Autodesk Inventor part; units mm, degrees
ref_plane "YZ Plane" through (0, 0, 0) normal (1, 0, 0) x (0, 1, 0)
ref_plane "XZ Plane" through (0, 0, 0) normal (0, 1, 0) x (-1, 0, 0)
ref_plane "XY Plane" through (0, 0, 0) normal (0, 0, 1) x (1, 0, 0)
sketch "Sketch1" plane through (0, 0, 0) normal (0, 0, 1) x (1, 0, 0)
  line L0 (0, 0) -> (20, 0)
  line L1 (20, 0) -> (20, 3.2)
  line L2 (0, 3.2) -> (20, 3.2)
  line L3 (0, 0) -> (0, 3.2)
  line L4 (20, -25) -> (0, -25)
  line L5 (0, -25) -> (0, -28.2)
  line L6 (20, -28.2) -> (0, -28.2)
  line L7 (20, -25) -> (20, -28.2)
  line L8 (3.2, -25) -> (3.2, 0)
  line L9 (0, -25) -> (0, 0)
  line L10 (-0.3, -0.3) -> (-0.3, 3.5)
  line L11 (-0.3, 3.5) -> (20.3, 3.5)
  line L12 (20.3, 3.5) -> (20.3, -0.3)
  line L13 (20.3, -24.7) -> (20.3, -28.5)
  line L14 (20.3, -28.5) -> (-0.3, -28.5)
  line L15 (-0.3, -28.5) -> (-0.3, -24.7)
  line L16 (3.5, -24.7) -> (3.5, -0.3)
  line L17 (-0.3, -0.3) -> (-0.3, -24.7)
  line L18 (20.3, -0.3) -> (3.5, -0.3)
  line L19 (3.5, -24.7) -> (20.3, -24.7)
  line L20 (6.5, -3.3) -> (6.5, -21.7)
  line L21 (6.5, -21.7) -> (23.3, -21.7)
  line L22 (23.3, -21.7) -> (23.3, -31.5)
  line L23 (23.3, -31.5) -> (-3.3, -31.5)
  line L24 (-3.3, -31.5) -> (-3.3, -24.7)
  line L25 (-3.3, -24.7) -> (-3.3, -0.3)
  line L26 (-3.3, -0.3) -> (-3.3, 6.5)
  line L27 (-3.3, 6.5) -> (23.3, 6.5)
  line L28 (23.3, 6.5) -> (23.3, -3.3)
  line L29 (23.3, -3.3) -> (6.5, -3.3)
  dimension "d2" = 0.3
  dimension "d3" = 0.3
  dimension "d4" = 0.3
  dimension "d5" = 24.4
  dimension "d6" = 3.8
  dimension "d7" = 3
extrude "Extrusion1" add sketch "Sketch1" against normal blind 15 contours L20 L21 L22 L23 L24 L25 L26 L27 L28 L29
sketch "Sketch4" plane through (0, 0, 0) normal (0, 0, 1) x (1, 0, 0)
  line L0 (23.3, -3.3) -> (23.3, 6.5)
  line L1 (23.3, 6.5) -> (-3.3, 6.5)
  line L2 (23.3, -3.3) -> (6.5, -3.3)
  line L3 (6.5, -3.3) -> (6.5, -21.7)
  line L4 (6.5, -21.7) -> (23.3, -21.7)
  line L5 (-3.3, -0.3) -> (-3.3, 6.5)
  line L6 (-3.3, -31.5) -> (23.3, -31.5)
  line L7 (23.3, -31.5) -> (23.3, -21.7)
  line L8 (23.3, -21.7) -> (6.5, -21.7)
  line L9 (23.3, 6.5) -> (23.3, -3.3)
  line L10 (23.3, -3.3) -> (23.3, 6.5)
  line L11 (-3.3, -31.5) -> (-3.3, 6.5)
  line L12 (23.3, 6.5) -> (-3.3, 6.5)
  line L13 (-3.3, 6.5) -> (-3.3, -31.5)
  line L14 (23.3, -31.5) -> (-3.3, -31.5)
  line L15 (-3.3, -31.5) -> (23.3, -31.5)
  line L16 (23.3, -21.7) -> (23.3, -31.5)
  line L17 (23.3, -31.5) -> (23.3, -21.7)
  line L18 (6.5, -3.3) -> (6.5, -21.7)
  line L19 (23.3, -3.3) -> (6.5, -3.3)
  line L20 (6.5, -3.3) -> (23.3, -3.3)
  line L21 (23.3, -3.3) -> (23.3, -21.7)
  point P0 (0, 0)
extrude "Extrusion3" add sketch "Sketch4" along normal blind 3
sketch "Sketch5" plane through (6.5, -21.7, -15) normal (1, 0, 0) x (0, 0, -1)
  line L0 (0, 18.4) -> (0, 0)
  line L1 (-15, 18.4) -> (0, 18.4)
  line L2 (-15, 0) -> (0, 0)
  line L3 (-15, 0) -> (-15, 18.4)
  circle A0 centre (-6, 9.2) radius 2
  circle A1 centre (-6, 9.2) radius 4
  point P0 (-15, 21.7)
  dimension "d14" = 4
  dimension "d15" = 6
  dimension "d16" = 8
  dimension "d17" = 9.2
extrude "Extrusion4" cut sketch "Sketch5" against normal blind 1 contours A1
extrude "Extrusion5" cut sketch "Sketch5" against normal blind 80 contours A0
sketch "Sketch16" plane through (-3.3, -31.5, -15) normal (-1, 0, 0) x (0, 0, 1)
  line L0 (18, 38) -> (18, 0)
  line L1 (0, 0) -> (18, 0)
  line L2 (18, 0) -> (18, 38)
  line L3 (18, 19) -> (0, 19) construction
  line L4 (0, 6.8) -> (0, 31.2)
  line L5 (18, 17.1) -> (18, 14.1)
  line L6 (18, 14.1) -> (9.94, 14.1)
  line L7 (9.94, 14.1) -> (9.94, 17.1)
  line L8 (9.94, 17.1) -> (18, 17.1)
  line L9 (18, 20.9) -> (18, 23.9)
  line L10 (18, 23.9) -> (9.94, 23.9)
  line L11 (9.94, 23.9) -> (9.94, 20.9)
  line L12 (9.94, 20.9) -> (18, 20.9)
  point P0 (15, 31.5)
  dimension "d41" = 3
  dimension "d42" = 1.9
  dimension "d43" = 8.06
extrude "Extrusion8" add sketch "Sketch16" along normal blind 20.03
fillet "Fillet1" radius 4 4 edges at (-23.33, -15.9, 3) (-23.33, -9.1, 3) (-23.33, -9.1, -5.06) (-23.33, -15.9, -5.06)
sketch "Sketch17" plane through (-3.3, -17.4, -5.06) normal (0, -1, 0) x (1, 0, 0)
  arc A0 (-16.03, 8.06) -> (-20.03, 4.06) centre (-16.03, 4.06) ccw
  circle A1 centre (-16.03, 4.06) radius 2.03
  point P0 (3.3, 5.06)
  dimension "d47" = 4.06
extrude "Extrusion9" cut sketch "Sketch17" against normal blind 20
properties part number "Tope_Carril"
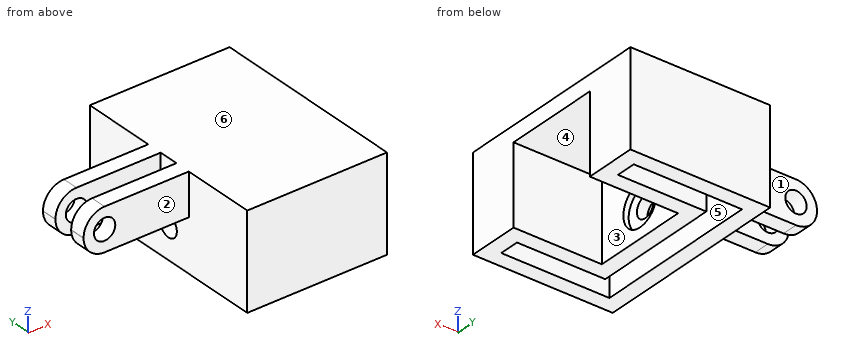
Could you check a few things on this model? Use its own coordinates, in mm. Face numbers are marked on the shaded views. A direction names the side the tool comes from. Coordinates: 2 decimals unless noted, no trailing zeros. Loops run counter-clockwise (first coordinate to the right, second up) from the corner with the lowest first, then second, coordinate; pieces in that order, holes last. Notation, with made-up numbers: (58, -17.5) -> (89, -17.5) arc R11 ccw to (89, -10.5) -> close; hole circle Ø9 at (-13.75, 11.5). An arc over 180 degrees is marked (long way). Answer in a Markdown table with one row per item.
(1) Imagine slicing it at C-C (y = -12.5). List the corners of the cut face in (x, z) for me, plus the area to 3 significant figures.
Results found:
| item | result |
|---|---|
| outline | (-3.3, -15) -> (-0.3, -15) -> (-0.3, -11) -> (-3.3, -11) -> close; (-3.3, -7) -> (-0.3, -7) -> (-0.3, 0) -> (3.5, 0) -> (3.5, -7) -> (5.5, -7) -> (5.5, -5) -> (6.5, -5) -> (6.5, 0) -> (23.3, 0) -> (23.3, 3) -> (-3.3, 3) -> close; (3.5, -15) -> (6.5, -15) -> (6.5, -13) -> (5.5, -13) -> (5.5, -11) -> (3.5, -11) -> close |
| area | 142 mm^2 |
(2) Thinking about a two-plate mould opening in Y: for the marked faces 1, 2 and 3, which applies, released by +Y, released by -Y, zero draft, split by the parting line, or undercut?
Results found:
| item | result |
|---|---|
| face 1 | released by +Y |
| face 2 | released by -Y |
| face 3 | undercut |
(3) Imagine slicing it at B-B (x = -10). List the corners of the cut face in (y, z) for me, plus the area to 3 significant figures.
Results found:
| item | result |
|---|---|
| outline | (-17.4, -5.06) -> (-14.4, -5.06) -> (-14.4, 3) -> (-17.4, 3) -> close; (-10.6, -5.06) -> (-7.6, -5.06) -> (-7.6, 3) -> (-10.6, 3) -> close |
| area | 48.4 mm^2 |
(4) Imagine slicing it at D-D (x = -18). List the corners of the cut face in (y, z) for me.
Results found:
| item | result |
|---|---|
| outline | (-17.4, -5.06) -> (-14.4, -5.06) -> (-14.4, -2.53) -> (-17.4, -2.53) -> close; (-17.4, 0.53) -> (-14.4, 0.53) -> (-14.4, 3) -> (-17.4, 3) -> close; (-10.6, -5.06) -> (-7.6, -5.06) -> (-7.6, -2.53) -> (-10.6, -2.53) -> close; (-10.6, 0.53) -> (-7.6, 0.53) -> (-7.6, 3) -> (-10.6, 3) -> close |
(5) Will these pins go through, and if not, where does the flat tip stop? pin 1 Ø10 at (y, z) = (-22, 1) entering from -X; pin 2 Ø6.5 at (x, z) = (-19.33, -1) entering from -Y; pin 3 Ø9 at (y, z) = (-12.5, -9) entering from +X; pin 4 Ø4.5 at (y, z) = (-12.5, -9) entering from +X.
Results found:
| item | result |
|---|---|
| pin 1 | stops at x = -23.33 |
| pin 2 | stops at y = -17.4 |
| pin 3 | stops at x = 6.5 |
| pin 4 | stops at x = 5.5 |
(6) If I drill on probe 1 along Y at (x, z) = (11, -11.25); probe 2 along X at (y, z) = (-2.5, -11.5); probe 3 along Y at (x, z) = (6, -3.25), over which ranges is the centre line in solid material (lowest first)?
Results found:
| item | result |
|---|---|
| probe 1 | y = -31.5 to -28.5, -24.7 to -21.7, -3.3 to -0.3, 3.5 to 6.5 |
| probe 2 | x = -3.3 to -0.3, 3.5 to 23.3 |
| probe 3 | y = -31.5 to -28.5, -24.7 to -0.3, 3.5 to 6.5 |
(7) For the marked faces 4, 5 and 6, which set-ups out of +Z, -Z, +X, -X, +Y, -Y let a thin tool reach every point of the face, with its end or its side?
Results found:
| item | result |
|---|---|
| face 4 | -Z, +X |
| face 5 | -Z |
| face 6 | +Z, +X, -X, +Y, -Y |
(8) Imagine slicing it at A-A (z = -9). List the corners of the cut face in (x, y) for me, plus the area to 3 significant figures.
Results found:
| item | result |
|---|---|
| outline | (-3.3, -31.5) -> (23.3, -31.5) -> (23.3, -21.7) -> (6.5, -21.7) -> (6.5, -16.5) -> (5.5, -16.5) -> (5.5, -14.5) -> (3.5, -14.5) -> (3.5, -24.7) -> (20.3, -24.7) -> (20.3, -28.5) -> (-0.3, -28.5) -> (-0.3, -14.5) -> (-3.3, -14.5) -> close; (-3.3, -10.5) -> (-0.3, -10.5) -> (-0.3, 3.5) -> (20.3, 3.5) -> (20.3, -0.3) -> (3.5, -0.3) -> (3.5, -10.5) -> (5.5, -10.5) -> (5.5, -8.5) -> (6.5, -8.5) -> (6.5, -3.3) -> (23.3, -3.3) -> (23.3, 6.5) -> (-3.3, 6.5) -> close |
| area | 424 mm^2 |
